Geometry: final body of the model. Coordinates: model frame, mm. Face numbers are marked on the shaded views. A direction names the side the tool comes from. Give positions to 0.01 mm unless a question says otherwise; leave off trailing zeros. Write each loop counter-clockwise with the first axis right and the second up, starting at its lowest first coordinate (ties: lowest second). Pieces come first, ordered by that corner, then holes. Notation, with made-up numbers: (-21.75, 42) - (-2.75, 42) arc R22 cw to (-2.75, 77) - close; hole circle Ø10 at (86, 22.5). An arc over 180 degrees is marked (long way). Use CSV: the item, a comma, the result in double quotes. Start each with the question number.
(1) Section B-B on x = 0. Output: boundary loops of the cut face in (y, z).
(2) Line query: probe 1 along X at (y, z) = (5.5, 0); probe 2 along Y at (x, z) = (-7, -1); probe 3 along Z at (x, y) = (-4.5, 8.75). Output: solid intervals per line, ascending. Write a range as [from, to].
(3) Reachability of the marked faces 4 and 5 from +Z, -Z, +X, -X, +Y, -Y: full face, straight path, thin tool, end or side. Return the list, or none.
(4) First-contact query: pin 1 Ø6 at (x, y) = (-10.5, 17.5) entering from +Z; pin 2 Ø3 at (x, z) = (7, -6.5) entering from +Y; pin 3 Ø3 at (x, z) = (-5.5, 13) entering from -Y. Flat tips, straight axial feed; report the tip coordinate or a pass-through.
(5) Section D-D on y = 13.75. Output: boundary loops of the cut face in (x, z).
(6) Section A-A on z = 0. Output: boundary loops of the cut face in (x, y), and give its area (3 significant figures).
(7) Section C-C on y = 6.25. Output: boundary loops of the cut face in (x, z), and give its area (3 significant figures).
(8) Draft query along X for the marked faces 1, 2 and 3. Return one class per face: released by +X, released by -X, zero draft, split by the parting line, or undercut.
from build123d import *

# Parameters (mm, degrees)
SKETCH2_R          = 6
CUT_EXTRUDE1_DEPTH = 33.156025874


with BuildPart() as part:
    # Sketch1 → Revolve1 (revolve)
    with BuildSketch(Plane.XY, mode=Mode.PRIVATE) as revolve1_sk:
        Polygon((17.4, 16.4), (12.132173, 20.7), (7.132173, 18), (5, 18), (5, 0), (12.5, 0), (12.5, 11.5), align=None)
    revolve(revolve1_sk.sketch.rotate(Axis((0, 20.7, 0), (0, -1, 0)), 270), axis=Axis((0, 20.7, 0), (0, -1, 0)))

    # Sketch2 → Cut-Extrude1 (cut, through all)
    with BuildSketch(Plane.XZ):
        with Locations(Location((0, 0, 0), (0, 0, 270))):
            Circle(SKETCH2_R)
    extrude(amount=-CUT_EXTRUDE1_DEPTH, mode=Mode.SUBTRACT)


solid = part.part
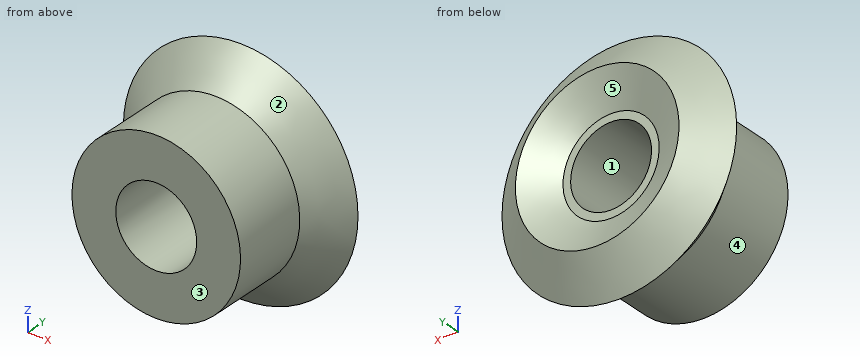
Check values:
1,outline,"(0, -12.5) - (11.5, -12.5) - (16.4, -17.4) - (20.7, -12.13) - (18, -7.13) - (18, -6) - (0, -6) - close; (0, 6) - (18, 6) - (18, 7.13) - (20.7, 12.13) - (16.4, 17.4) - (11.5, 12.5) - (0, 12.5) - close"
2,probe 1,"x = [-12.5, -6], [6, 12.5]"
2,probe 2,"y = [0, 18]"
2,probe 3,"z = [-11.66, -3.97], [3.97, 11.66]"
3,face 4,"-Y"
3,face 5,"+Y"
4,pin 1,"stops at z = 15.6"
4,pin 2,"stops at y = 20.12"
4,pin 3,"stops at y = 11.62"
5,outline,"circle Ø29.5 at (0, 0); hole circle Ø12 at (0, 0)"
6,outline,"(-17.4, 16.4) - (-12.5, 11.5) - (-12.5, 0) - (-6, 0) - (-6, 18) - (-7.13, 18) - (-12.13, 20.7) - close; (6, 0) - (12.5, 0) - (12.5, 11.5) - (17.4, 16.4) - (12.13, 20.7) - (7.13, 18) - (6, 18) - close"
6,area,"293 mm²"
7,outline,"circle Ø25 at (0, 0); hole circle Ø12 at (0, 0)"
7,area,"378 mm²"
8,face 1,"undercut"
8,face 2,"split by the parting line"
8,face 3,"zero draft"
